Model file for the job. Use its own axes, mm. Face numbers are marked on the shaded views. A direction names the side the tool comes from. Coordinates: 2 decimals unless noted, no trailing zeros. Write each loop counter-clockwise with the first axis right and the second up, starting at its lowest first coordinate (ties: lowest second). Pieces come first, ordered by that corner, then holes. Notation, with made-up numbers: (8, -21) -> (17, -21) arc R20 cw to (17, -10) -> close; hole circle Ø11 at (-39.5, -5). An arc over 180 degrees is marked (long way). Write item = value, one per line. Start each with the question number.
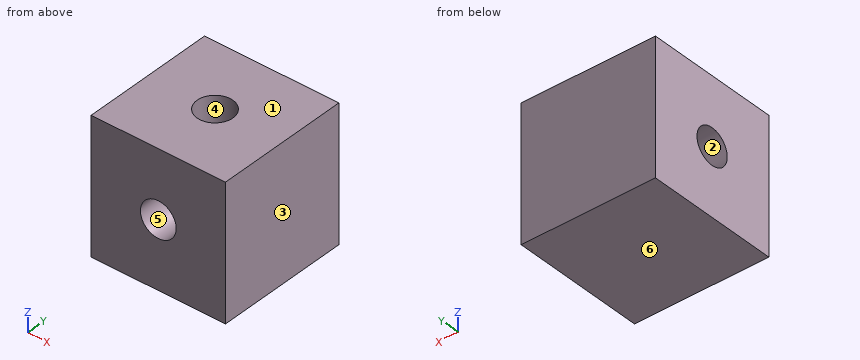
from build123d import *

# Parameters (mm, degrees)
F0_W     = 19.05
F0_H     = 19.05
F1_DEPTH = 19.05
F3_D     = 5.08
F3_DEPTH = 6.35
F3_TIP   = 1.5261859723
F5_D     = 5.08
F5_DEPTH = 6.35
F5_TIP   = 1.5261859723
F7_D     = 5.08
F7_DEPTH = 6.35
F7_TIP   = 1.5261859723


with BuildPart() as f1:
    # F0 (on Top) → F1 (new body)
    with BuildSketch(Plane.XY):
        Rectangle(F0_W, F0_H)
    extrude(amount=F1_DEPTH)

    # F3
    with Locations(Plane.XZ.offset(9.525)):
        with Locations((0, 9.525)):
            Hole(F3_D / 2, depth=F3_DEPTH)
            with Locations((0, 0, -(F3_DEPTH + F3_TIP / 2))):  # 118° drill point
                Cone(0, F3_D / 2, F3_TIP, mode=Mode.SUBTRACT)

    # F5
    with Locations(Plane(origin=(-9.525, 0, 0), x_dir=(0, -1, 0), z_dir=(-1, 0, 0))):
        with Locations((0, 9.525)):
            Hole(F5_D / 2, depth=F5_DEPTH)
            with Locations((0, 0, -(F5_DEPTH + F5_TIP / 2))):  # 118° drill point
                Cone(0, F5_D / 2, F5_TIP, mode=Mode.SUBTRACT)

    # F7
    with Locations(Plane.XY.offset(19.05)):
        with Locations((0, 0)):
            Hole(F7_D / 2, depth=F7_DEPTH)
            with Locations((0, 0, -(F7_DEPTH + F7_TIP / 2))):  # 118° drill point
                Cone(0, F7_D / 2, F7_TIP, mode=Mode.SUBTRACT)


solid = f1.part
(1) Saw through at B-B (z = 14.5). Give the cut face in (x, y) (3 decimals).
(2) Mould opens along X. For the marked faces 3, 4, 5 and 6 say: released by +X, released by -X, zero draft, split by the parting line, or undercut.
(3) Drill centre lines: line 1 along Z through (x, y) = (-6.5, 0) (3 decimals); line 2 along Y through (x, z) = (0, 14.75) (3 decimals); line 3 along X through (y, z) = (-7.75, 10.75) (3 decimals). Where is each one in solid material? Low to high.
(4) 3-axis set-ups, long thin cutter, end or side, ignore diameter. For the marked faces 1 and 2: which of +Z, -Z, +X, -X, +Y, -Y reach the whole face in a straight line?
(5) Saw through at A-A (y = -5.75). Give the cut face in (x, z) (3 decimals), then the cut area to 3 significant figures.
(6) Drop a flat-ended pin along its axis: pin 1 Ø3 at (x, y) = (0, -2) entering from -Z. Give the stop position or say it passes through.
Returned:
q1.outline = (-9.525, -9.525) -> (9.525, -9.525) -> (9.525, 9.525) -> (-9.525, 9.525) -> close; hole circle Ø5.08 at (0, 0)
q2.face_3 = released by +X
q2.face_4 = undercut
q2.face_5 = undercut
q2.face_6 = zero draft
q3.line_1 = 0 to 6.985, 12.065 to 19.05
q3.line_2 = -9.525 to -2.54, 2.54 to 9.525
q3.line_3 = -9.525 to -2.225, 2.225 to 9.525
q4.face_1 = +Z, +X, -X, +Y, -Y
q4.face_2 = -X
q5.outline = (-9.525, 0) -> (9.525, 0) -> (9.525, 19.05) -> (-9.525, 19.05) -> close; hole circle Ø5.08 at (0, 9.525)
q5.area = 343 mm2
q6.pin_1 = 0
